The model under review builds one solid part; all positions refer to its coordinate system, in mm. Face numbers are marked on the shaded views. A direction names the side the tool comes from. Coordinates: 2 decimals unless noted, no trailing zeros. Loops run counter-clockwise (first coordinate to the right, second up) from the corner with the lowest first, then second, coordinate; pieces in that order, holes last. Notation, with made-up numbers: (-34.75, 9) - (-28.75, 9) arc R21 cw to (-28.75, 32) - close; hole circle Ø5 at (64.5, -4.5). An arc over 180 degrees is marked (long way). One line per item, written item: value. Start each with the question number.
1. Mouldability with a two-part tool opening along X and no side actions: class the marked faces 3, 4 and 5 as +X half, -X half, draft (parallel to the pull), parting line (faces both ways), or undercut.
2. We need section B-B, the plane z = 16.5. Give the boundary of the cut face in (x, y).
3. For the marked faces 1 and 2, list the 3-axis set-ups (+Z, -Z, +X, -X, +Y, -Y) from which the entire face can be reached by the end or side of a thin tool; tool diameter is ignored.
4. To check wall thickness, follow line 1 (Y direction, x = -2, z = 21); line 2 (X direction, y = -4.5, z = 3.5); line 3 (Z direction, x = -14, y = -5.5). State the ranges of each line that lie inside material, in increasing order.
5. We need section C-C, the plane y = -6. Give the boundary of the cut face in (x, z), then the cut area to 3 significant figures.
6. Insertion check: P1, Ø1.1, axis at y = 9, z = 35.5, coming from the -X side; P2, Ø0.5, axis at y = -9, z = 35, coming from the +X side; P3, Ø1, axis at x = -2.5, y = -1.5, coming from the +Z side. Each pin has a flat end and moves straight along its axis. Give the tip position at first contact, or say it passes through.
7. We need section D-D, the plane x = 7. Give the boundary of the cut face in (y, z).
8. We need section A-A, the plane z = 35.5. Give the boundary of the cut face in (x, y).
Solid Edge part; units mm, degrees
sketch "Sketch1" plane through (0, 0, 0) normal (0, 0, 1) x (1, 0, 0)
  arc A0 (-15.5424, 9.5) -> (-15.5424, -9.5) centre (-1.4446, 0) ccw
  line L0 (-15.5424, -9.5) -> (15.5424, -9.5)
  arc A1 (15.5424, -9.5) -> (15.5424, 9.5) centre (1.4446, 0) ccw
  line L1 (15.5424, 9.5) -> (-15.5424, 9.5)
extrude "Protrusion1" add sketch "Sketch1" against normal blind 1
sketch "Sketch2" plane through (0, 0, 0) normal (0, 0, 1) x (1, 0, 0)
  arc A0 (-15.5424, 9.5) -> (-15.5424, -9.5) centre (-1.4446, 0) ccw
  line L0 (-15.5424, -9.5) -> (15.5424, -9.5)
  arc A1 (15.5424, -9.5) -> (15.5424, 9.5) centre (1.4446, 0) ccw
  line L1 (15.5424, 9.5) -> (-15.5424, 9.5)
  line L2 (-15, -8.5) -> (15, -8.5)
  arc A2 (15, 8.5) -> (15, -8.5) centre (1.4446, 0) cw
  line L3 (15, 8.5) -> (-15, 8.5)
  arc A3 (-15, 8.5) -> (-15, -8.5) centre (-1.4446, 0) ccw
extrude "ProtrusioneEstrusa_2" add sketch "Sketch2" along normal blind 40
sketch "Sketch3" plane through (0, -9.5, 19.5) normal (0, -1, 0) x (1, 0, 0)
  line L0 (2.5, 14.25) -> (2.5, 16.75)
  line L1 (2.5, 16.75) -> (-2.5, 16.75)
  line L2 (-2.5, 16.75) -> (-2.5, 14.25)
  line L3 (-2.5, 14.25) -> (2.5, 14.25)
extrude "ScavoEstrusione_1" cut sketch "Sketch3" along normal mid plane 58.0417
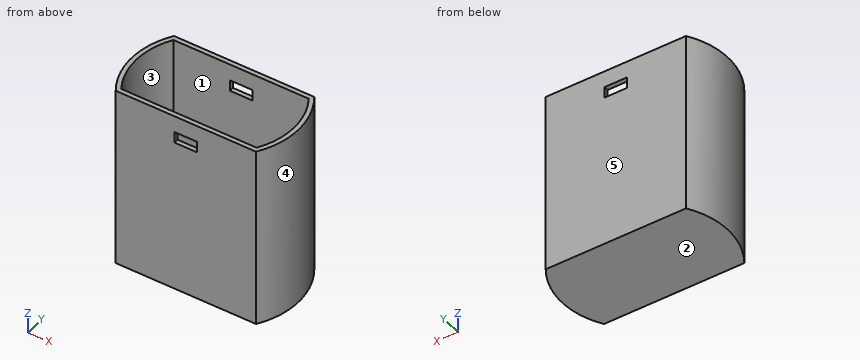
Findings below:
1. face 3: undercut
1. face 4: +X half
1. face 5: draft
2. outline: (-15.54, -9.5) - (15.54, -9.5) arc R17 ccw to (15.54, 9.5) - (-15.54, 9.5) arc R17 ccw to start; hole (-15, -8.5) - (15, -8.5) arc R16 ccw to (15, 8.5) - (-15, 8.5) arc R16 ccw to start
3. face 1: +Z
3. face 2: -Z, +X, -X, +Y, -Y
4. line 1: -9.5 to -8.5, 8.5 to 9.5
4. line 2: -17.84 to -16.8, 16.8 to 17.84
4. line 3: -1 to 0
5. outline: (-17.35, -1) - (17.35, -1) - (17.35, 40) - (16.28, 40) - (16.28, 0) - (-16.28, 0) - (-16.28, 40) - (-17.35, 40) - close
5. area: 121 mm2
6. P1: x = -16.2
6. P2: x = 16.02
6. P3: z = 0
7. outline: (-9.5, -1) - (9.5, -1) - (9.5, 40) - (8.5, 40) - (8.5, 0) - (-8.5, 0) - (-8.5, 40) - (-9.5, 40) - close
8. outline: (-15.54, -9.5) - (-2.5, -9.5) - (-2.5, -8.5) - (-15, -8.5) arc R16 cw to (-15, 8.5) - (-2.5, 8.5) - (-2.5, 9.5) - (-15.54, 9.5) arc R17 ccw to start; (2.5, -9.5) - (15.54, -9.5) arc R17 ccw to (15.54, 9.5) - (2.5, 9.5) - (2.5, 8.5) - (15, 8.5) arc R16 cw to (15, -8.5) - (2.5, -8.5) - close
